Read the model definition and answer for the solid it produces. Units are mm, in the model's axes. Face numbers are marked on the shaded views. A direction names the side the tool comes from. Coordinates: 2 decimals unless noted, no trailing zeros. Loops run counter-clockwise (first coordinate to the right, second up) from the corner with the lowest first, then second, coordinate; pieces in that order, holes last. Notation, with made-up numbers: M 35.25,14.25 L 59.25,14.25 A8 cw 59.25,29.25 Z; hole C 49.5,54.25 d5. An arc over 180 degrees is marked long. One line per item, written item: value. Start each with the question number.
1. The part is cut by section D-D (y = -6.5). Write down the section's boundary in (x, z), then the cut area to 3 significant figures.
2. The part is cut by section C-C (x = -1.3). Write down the section's boundary in (y, z), then the cut area to 3 significant figures.
3. The part is cut by section B-B (z = -1.15). Write down the section's boundary in (x, y).
4. Determine the mould class of the marked faces 3, 4 and 5 for opening direction Z: +Z half, -Z half, draft (parallel to the pull), parting line (faces both ways), or undercut.
5. For the marked faces 1 and 2, determine the directions among +Z, -Z, +X, -X, +Y, -Y from which every point of the face is accessible in a straight line to the end or side of a thin tool.
6. Consider probe 1 along X at (y, z) = (-2.75, 1.6); probe 2 along X at (y, z) = (-3.25, -0.4); probe 3 along X at (y, z) = (-1.25, -0.8). Determine where each line is inside the solid, lowest interval first.
7. A flat-ended cylindrical pin translates along its axis: pin 1 (1.5 mm diameter, centred on y = -7, z = 1.5, fed in from -X). Find the tip coordinate at first contact, or state that the pin passes through.
8. The part is cut by section A-A (y = -0.5). State how many separate pieces and enclosed holes the cut face has, then the cut area to 3 significant figures.
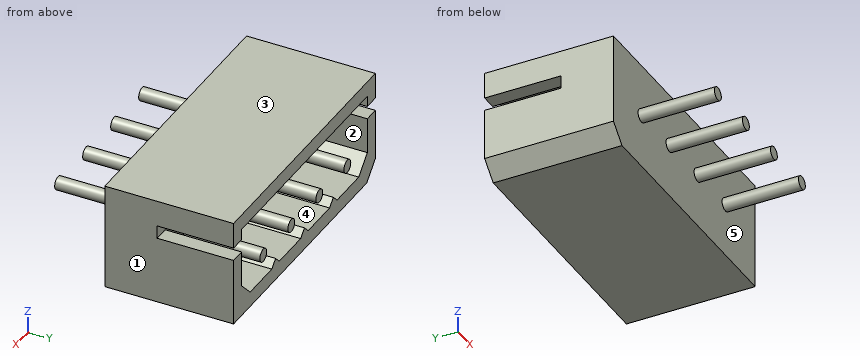
```python
from build123d import *

# Parameters (mm, degrees)
BOSS_EXTRUDE1_DEPTH = 5.9
SKETCH2_R           = 0.3
BOSS_EXTRUDE2_DEPTH = 3.5
SKETCH3_R           = 0.3
CUT_EXTRUDE1_DEPTH  = 3.5


with BuildPart() as part:
    # Sketch1 → Boss-Extrude1 (new body)
    with BuildSketch(Plane(origin=(0, 0, 0), x_dir=(1, 0, 0), z_dir=(0, 1, 0))):
        Polygon((-5.45, 2.45), (-6.2, 1.7), (-6.2, -2.45), (6.2, -2.45), (6.2, 2.45), align=None)
    extrude(amount=-BOSS_EXTRUDE1_DEPTH)

    # Sketch2 → Boss-Extrude2 (add)
    with BuildSketch(Plane.XZ.offset(5.9)):
        with Locations(Location((-3.75, 0, 0), (0, 0, 90))):
            Circle(SKETCH2_R)
        with Locations(Location((-1.3, 0, 0), (0, 0, 90))):
            Circle(SKETCH2_R)
        with Locations(Location((1.15, 0, 0), (0, 0, 90))):
            Circle(SKETCH2_R)
        with Locations(Location((3.6, 0, 0), (0, 0, 90))):
            Circle(SKETCH2_R)
    extrude(amount=BOSS_EXTRUDE2_DEPTH)

    # Sketch3 → Cut-Extrude1 (cut)
    with BuildSketch(Plane(origin=(0, 0, 0), x_dir=(1, 0, 0), z_dir=(0, 1, 0))):
        Polygon((-2.853247496, 1.75), (-4.75, 1.75), (-5.5, 1), (-5.5, -0.65), (-6.2, -0.65), (-6.2, -1.25), (-5.5, -1.25), (-5.5, -1.75), (5.5, -1.75), (5.5, -1.25), (6.2, -1.25), (6.2, -0.65), (5.5, -0.65), (5.5, 1), (4.75, 1.75), (2.853247496, 1.75), (2.525, 1.421752504), (2.196752504, 1.75), (0.328247496, 1.75), (0, 1.421752504), (-0.328247496, 1.75), (-2.196752504, 1.75), (-2.525, 1.421752504), align=None)
        with Locations(Location((-3.75, 0.63, 0), (0, 0, 270))):
            Circle(SKETCH3_R, mode=Mode.SUBTRACT)
        with Locations(Location((-1.3, 0.63, 0), (0, 0, 270))):
            Circle(SKETCH3_R, mode=Mode.SUBTRACT)
        with Locations(Location((1.15, 0.63, 0), (0, 0, 270))):
            Circle(SKETCH3_R, mode=Mode.SUBTRACT)
        with Locations(Location((3.6, 0.63, 0), (0, 0, 270))):
            Circle(SKETCH3_R, mode=Mode.SUBTRACT)
    extrude(amount=-CUT_EXTRUDE1_DEPTH, mode=Mode.SUBTRACT)


solid = part.part
```
Answer block:
1. outline: C -3.75,0 d0.6; C -1.3,0 d0.6; C 1.15,0 d0.6; C 3.6,0 d0.6
1. area: 1.13 mm2
2. outline: M -9.4,-0.3 L -5.9,-0.3 L -5.9,-2.45 L 0,-2.45 L 0,-1.75 L -3.5,-1.75 L -3.5,-0.93 L 0,-0.93 L 0,-0.33 L -3.5,-0.33 L -3.5,1.75 L 0,1.75 L 0,2.45 L -5.9,2.45 L -5.9,0.3 L -9.4,0.3 Z
2. area: 20.9 mm2
3. outline: M -6.2,-5.9 L 6.2,-5.9 L 6.2,0 L 5.35,0 L 5.35,-3.5 L -5.35,-3.5 L -5.35,0 L -6.2,0 Z
4. face 3: +Z half
4. face 4: undercut
4. face 5: draft
5. face 1: +Z, -Z, +X, +Y, -Y
5. face 2: +Y
6. probe 1: x = -6.2 to -5.5, 5.5 to 6.2
6. probe 2: x = -6.2 to -5.5, -3.94 to -3.56, -1.49 to -1.11, 0.96 to 1.34, 3.41 to 3.79, 5.5 to 6.2
6. probe 3: x = -6.2 to -5.5, -4 to -3.5, -1.55 to -1.05, 0.9 to 1.4, 3.35 to 3.85, 5.5 to 6.2
7. pin 1: passes through
8. separate pieces: 6
8. enclosed holes: 0
8. area: 23.2 mm2
